from build123d import *

# Parameters (mm, degrees)
SKETCH1_W               = 55
SKETCH1_H               = 42.5
BOSS_EXTRUDE1_DEPTH     = 23.5
CUT_EXTRUDE1_DEPTH      = 64.4729273
CUT_EXTRUDE1_DEPTH_BACK = 64.4729273
CUT_EXTRUDE2_DEPTH      = 42.953098813
CUT_EXTRUDE2_DEPTH_BACK = 42.953098813
CUT_EXTRUDE3_DEPTH      = 42.953098813
CUT_EXTRUDE3_DEPTH_BACK = 42.953098813
SKETCH4_W               = 23
SKETCH4_H               = 12.5
CUT_EXTRUDE4_DEPTH      = 42.978446851
CUT_EXTRUDE4_DEPTH_BACK = 42.978446851
SKETCH5_R               = 1.575
BOSS_EXTRUDE2_DEPTH     = 2
BOSS_EXTRUDE3_DEPTH     = 2
BOSS_EXTRUDE4_DEPTH     = 2
SKETCH11_R              = 1.55
CUT_EXTRUDE5_DEPTH      = 2


with BuildPart() as part:
    # Sketch1 → Boss-Extrude1 (new body)
    with BuildSketch(Plane.XY):
        Rectangle(SKETCH1_W, SKETCH1_H)
    extrude(amount=BOSS_EXTRUDE1_DEPTH)

    # Sketch2 → Cut-Extrude1 (cut, two sides: drawn at the far end of the back side and taken through both)
    with BuildSketch(Plane(origin=(27.5, 0, 0), x_dir=(0, 0, -1), z_dir=(1, 0, 0)).offset(-CUT_EXTRUDE1_DEPTH_BACK)):
        with BuildLine():
            Line((-3, 21.25), (-3, 8.95))
            Line((-3, 8.95), (-11, 8.95))
            Line((-11, 8.95), (-11, -0.05))
            Line((-11, -0.05), (-23.5, -0.05))
            Line((-23.5, -0.05), (-23.5, -3.05))
            Line((-23.5, -3.05), (-9.5, -3.05))
            ThreePointArc((-9.5, -3.05), (-8.085786438, -3.635786438), (-7.5, -5.05))
            Line((-7.5, -5.05), (-7.5, -12.05))
            Line((-7.5, -12.05), (-5.5, -10.55))
            Line((-5.5, -10.55), (-2.5, -10.55))
            Line((-2.5, -10.55), (-2.5, -17.55))
            Line((-2.5, -17.55), (-5.5, -17.55))
            Line((-5.5, -17.55), (-7.5, -16.05))
            Line((-7.5, -16.05), (-7.5, -21.25))
            Line((-7.5, -21.25), (-33.241676539, -21.25))
            Line((-33.241676539, -21.25), (-33.241676539, 21.25))
            Line((-33.241676539, 21.25), (-3, 21.25))
        make_face()
    extrude(amount=CUT_EXTRUDE1_DEPTH + CUT_EXTRUDE1_DEPTH_BACK, mode=Mode.SUBTRACT)

    # Sketch3 → Cut-Extrude2 (cut, two sides: drawn at the far end of the back side and taken through both)
    with BuildSketch(Plane(origin=(0, 0, 0), x_dir=(1, 0, 0), z_dir=(0, 1, 0)).offset(-CUT_EXTRUDE2_DEPTH_BACK)):
        Polygon((7.5, -10.995887084), (7.5, -23.5), (27.5, -23.5), (27.5, -10.993542952), (27.5, -7.5), (7.5, -7.5), align=None)
    extrude(amount=CUT_EXTRUDE2_DEPTH + CUT_EXTRUDE2_DEPTH_BACK, mode=Mode.SUBTRACT)

    # Sketch4 → Cut-Extrude3 (cut, two sides: drawn at the far end of the back side and taken through both)
    with BuildSketch(Plane(origin=(0, 0, 0), x_dir=(1, 0, 0), z_dir=(0, 1, 0)).offset(-CUT_EXTRUDE3_DEPTH_BACK)):
        with Locations((-10, -17.25)):
            Rectangle(SKETCH4_W, SKETCH4_H)
    extrude(amount=CUT_EXTRUDE3_DEPTH + CUT_EXTRUDE3_DEPTH_BACK, mode=Mode.SUBTRACT)

    # Sketch5 → Cut-Extrude4 (cut, two sides: drawn at the far end of the back side and taken through both)
    with BuildSketch(Plane(origin=(0, -0.05, 0), x_dir=(1, 0, 0), z_dir=(0, 1, 0)).offset(-CUT_EXTRUDE4_DEPTH_BACK)):
        with Locations(Location((-24.5, -17.25, 0), (0, 0, 270))):
            Circle(SKETCH5_R)
        with Locations(Location((4.5, -17.25, 0), (0, 0, 270))):
            Circle(SKETCH5_R)
    extrude(amount=CUT_EXTRUDE4_DEPTH + CUT_EXTRUDE4_DEPTH_BACK, mode=Mode.SUBTRACT)

    # Sketch6 → Boss-Extrude2 (add)
    with BuildSketch(Plane(origin=(0, 21.25, 0), x_dir=(1, 0, 0), z_dir=(0, 1, 0))):
        with BuildLine():
            Line((-27.5, -3), (-27.5, -16))
            Line((-27.5, -16), (-20.5, -16))
            ThreePointArc((-20.5, -16), (-16.964466094, -14.535533906), (-15.5, -11))
            Line((-15.5, -11), (-15.5, -3))
            Line((-15.5, -3), (-27.5, -3))
        make_face()
        with BuildLine():
            Line((15.5, -3), (27.5, -3))
            Line((27.5, -3), (27.5, -16))
            Line((27.5, -16), (20.5, -16))
            ThreePointArc((20.5, -16), (16.964466094, -14.535533906), (15.5, -11))
            Line((15.5, -11), (15.5, -3))
        make_face()
    extrude(amount=-BOSS_EXTRUDE2_DEPTH)

    # Sketch7 → Boss-Extrude3 (add)
    with BuildSketch(Plane(origin=(27.5, 0, 0), x_dir=(0, 0, -1), z_dir=(1, 0, 0))):
        Polygon((-3, 19.25), (-3, 10.150500969), (-16, 19.25), align=None)
    extrude(amount=-BOSS_EXTRUDE3_DEPTH)

    # Sketch9 → Boss-Extrude4 (add)
    with BuildSketch(Plane.ZY.offset(27.5)):
        Polygon((16, 19.25), (3, 10.150500969), (3, 19.25), align=None)
    extrude(amount=-BOSS_EXTRUDE4_DEPTH)

    # Sketch11 → Cut-Extrude5 (cut)
    with BuildSketch(Plane(origin=(0, 21.25, 0), x_dir=(1, 0, 0), z_dir=(0, 1, 0))):
        with Locations(Location((-20.5, -9.5, 0), (0, 0, 180))):
            Circle(SKETCH11_R)
        with Locations(Location((20.5, -9.5, 0), (0, 0, 180))):
            Circle(SKETCH11_R)
    extrude(amount=-CUT_EXTRUDE5_DEPTH, mode=Mode.SUBTRACT)


solid = part.part
Can you work these out from the model? Positions are in its coordinate system, mm. A direction names the side the tool comes from. Coordinates: 2 decimals unless noted, no trailing zeros. Loops run counter-clockwise (first coordinate to the right, second up) from the corner with the lowest first, then second, coordinate; pieces in that order, holes last. Notation, with made-up numbers: M 83,2 L 120,2 A19 ccw 120,26 Z; hole C 67.5,-15.75 d10. An arc over 180 degrees is marked long. Return JSON: item names as keys, results as strings. Group by question number.
Item 1: If I drill on L1, parallel to X at y = -0.7, z = 17.25 (3 decimals); L2, parallel to Y at x = 20.5, z = 2.75; L3, parallel to Y at x = 3, z = 19, over which ranges is the centre line in solid material (lowest first)? Write a range as from..to.
Item 2: I'm going to push flat-ended pins straight in: pin 1 Ø7.5 at (x, y) = (12, -15) entering from +Z; pin 2 Ø5 at (x, z) = (19.5, 14.5) entering from -Y; pin 3 Ø17 at (x, y) = (5, 1.5) entering from +Z; pin 4 Ø6.5 at (x, z) = (6, 19.5) entering from +Y. Where does each tip first touch, or does it pass through?
Item 3: Imagine slicing it at A-A (x = -24.5). Please give me the cut outline in (y, z) (3 decimals), and give its area (3 significant figures).
Item 4: Imagine slicing it at C-C (y = 17.5). Please give me the cut outline in (x, z).
Item 5: Thinking about a two-plate mould opening in Y: for faces 1 (the flat face through (-0.4, 21.25, 2.6)), 2 (the flat face through (-0.4, -11.3, 6.5)), 3 (the flat face through (7.5, -1, 14)), 4 (the flat face through (-26.514, 14.764, 9.591)), which applies, released by +Y, released by -Y, zero draft, split by the parting line, or undercut?
Item 6: On a 3-axis mill with a long thin cutter (end or side, diameter ignored), from which of +Z, -Z, +X, -X, +Y, -Y can I reach the whole of each face in a straight line? I mean faces 5 (the cylindrical face through (-21.932, 20.264, 8.906)), 6 (the flat face through (0, -19, 7.5)), 7 (the flat face through (-22, 19.25, 8)), 8 (the flat face through (0, -10.55, 4)). Say none if no direction works.
Item 7: Imagine slicing it at D-D (x = 14). Please give me the cut outline in (y, z), and give its area (3 significant figures).
Item 8: Imagine slicing it at B-B (x = -9.5). Please give me the cut outline in (y, z).
Verdict:
{
 "1": {"L1": "x = -27.5..-26.075, -22.925..-21.5, 1.5..2.925, 6.075..7.5", "L2": "y = -21.25..-17.55, -10.55..21.25", "L3": "y = -3.05..-0.05"},
 "2": {"pin 1": "stops at z = 7.5", "pin 2": "stops at y = 19.25", "pin 3": "stops at z = 23.5", "pin 4": "stops at y = -0.05"},
 "3": {"outline": "M -21.25,0 L 21.25,0 L 21.25,16 L 19.25,16 L 19.25,3 L 8.95,3 L 8.95,11 L -0.05,11 L -0.05,15.675 L -3.05,15.675 L -3.05,9.5 A2 cw -5.05,7.5 L -12.05,7.5 L -10.55,5.5 L -10.55,2.5 L -17.55,2.5 L -17.55,5.5 L -16.05,7.5 L -21.25,7.5 Z; M -3.05,18.825 L -0.05,18.825 L -0.05,23.5 L -3.05,23.5 Z", "area": "328 mm^2"},
 "4": {"outline": "M -27.5,0 L 27.5,0 L 27.5,13.5 L 25.5,13.5 L 25.5,3 L -25.5,3 L -25.5,13.5 L -27.5,13.5 Z"},
 "5": {"face 1": "released by +Y", "face 2": "undercut", "face 3": "zero draft", "face 4": "undercut"},
 "6": {"face 5": "+Y", "face 6": "+Z, +X, -X, -Y", "face 7": "+Z", "face 8": "+X, -X"},
 "7": {"outline": "M -21.25,0 L 21.25,0 L 21.25,3 L 8.95,3 L 8.95,7.5 L -12.05,7.5 L -10.55,5.5 L -10.55,2.5 L -17.55,2.5 L -17.55,5.5 L -16.05,7.5 L -21.25,7.5 Z", "area": "231 mm^2"},
 "8": {"outline": "M -21.25,0 L 21.25,0 L 21.25,3 L 8.95,3 L 8.95,11 L -3.05,11 L -3.05,9.5 A2 cw -5.05,7.5 L -12.05,7.5 L -10.55,5.5 L -10.55,2.5 L -17.55,2.5 L -17.55,5.5 L -16.05,7.5 L -21.25,7.5 Z"}
}
